from build123d import *

# Parameters (mm, degrees)
SKETCH_3_R                         = 2.75
EXTRUDE_1_DEPTH                    = 2
PATTERN_CIRCULAR_1_COUNT           = 4
SKETCH_7_R                         = 1.5
CUT_EXTRUDE_3_DEPTH                = 10
CUT_EXTRUDE_4_DEPTH                = 3
PATTERN_CIRCULAR_3_COUNT           = 3
PATTERN_CIRCULAR_3_ANGLE           = 60
PATTERN_CIRCULAR_4_COUNT           = 4
PATTERN_CIRCULAR_4_COPY_1_SKETCH_R = 1.5
PATTERN_CIRCULAR_4_COPY_1_DEPTH    = 10
PATTERN_CIRCULAR_4_COPY_2_SKETCH_R = 1.5
PATTERN_CIRCULAR_4_COPY_2_DEPTH    = 10
PATTERN_CIRCULAR_4_COPY_3_SKETCH_R = 1.5
PATTERN_CIRCULAR_4_COPY_3_DEPTH    = 10
PATTERN_CIRCULAR_4_COPY_4_SKETCH_R = 1.5
PATTERN_CIRCULAR_4_COPY_4_DEPTH    = 10
PATTERN_CIRCULAR_4_COPY_5_SKETCH_R = 1.5
PATTERN_CIRCULAR_4_COPY_5_DEPTH    = 10
PATTERN_CIRCULAR_4_COPY_6_SKETCH_R = 1.5
PATTERN_CIRCULAR_4_COPY_6_DEPTH    = 10
PATTERN_CIRCULAR_4_COPY_7_DEPTH    = 3
PATTERN_CIRCULAR_4_COPY_8_DEPTH    = 3
PATTERN_CIRCULAR_4_COPY_9_DEPTH    = 3
PATTERN_CIRCULAR_4_COPY_10_DEPTH   = 3
PATTERN_CIRCULAR_4_COPY_11_DEPTH   = 3
PATTERN_CIRCULAR_4_COPY_12_DEPTH   = 3
FILLET_1_R                         = 0.5


with BuildPart() as part:
    # 草图2 → 旋转1 (revolve)
    with BuildSketch(Plane(origin=(0, 0, 0), x_dir=(1, 0, 0), z_dir=(0, 1, 0)), mode=Mode.PRIVATE) as revolve_1_sk:
        Polygon((0, -2.5), (30, -2.5), (27.5, 0), (30, 2.5), (0, 2.5), align=None)
    revolve(revolve_1_sk.sketch.rotate(Axis((0, 0, -2.5), (0, 0, 1)), 180), axis=Axis((0, 0, -2.5), (0, 0, 1)))

    # 草图3 → 凸台-拉伸1 (add)
    with BuildSketch(Plane.XY.offset(2.5)):
        with Locations(Location((4.788152334, 17.869627786, 0), (0, 0, 180))):
            Circle(SKETCH_3_R)
    extrude_1 = extrude(amount=EXTRUDE_1_DEPTH)

    # 阵列(圆周)1: 凸台-拉伸1 ×4 about axis
    pattern_circular_1_axis = Axis((0, 0, 0), (0, 0, 1))
    for i in range(1, PATTERN_CIRCULAR_1_COUNT):
        add(extrude_1.rotate(pattern_circular_1_axis, i * 360 / PATTERN_CIRCULAR_1_COUNT))

    # 草图7 → 切除-拉伸3 (cut)
    with BuildSketch(Plane(origin=(0, 0, -2.5), x_dir=(-1, 0, 0), z_dir=(0, 0, -1))):
        with Locations((4.788152334, 17.869627786)):
            Circle(SKETCH_7_R)
    cut_extrude_3 = extrude(amount=-CUT_EXTRUDE_3_DEPTH, mode=Mode.SUBTRACT)

    # 草图8 → 切除-拉伸4 (cut)
    with BuildSketch(Plane(origin=(0, 0, -2.5), x_dir=(-1, 0, 0), z_dir=(0, 0, -1))):
        Polygon((3.966291485, 14.802401339), (7.033517932, 15.624262189), (7.855378781, 18.691488636), (5.610013184, 20.936854233), (2.542786737, 20.114993384), (1.720925887, 17.047766937), align=None)
    cut_extrude_4 = extrude(amount=-CUT_EXTRUDE_4_DEPTH, mode=Mode.SUBTRACT)

    # 阵列(圆周)3: 切除-拉伸3, 切除-拉伸4 ×3 about axis
    pattern_circular_3_axis = Axis((0, 0, 0), (0, 0, 1))
    add([cut_extrude_3.rotate(pattern_circular_3_axis, i * PATTERN_CIRCULAR_3_ANGLE / (PATTERN_CIRCULAR_3_COUNT - 1)) for i in range(1, PATTERN_CIRCULAR_3_COUNT)], mode=Mode.SUBTRACT)
    add([cut_extrude_4.rotate(pattern_circular_3_axis, i * PATTERN_CIRCULAR_3_ANGLE / (PATTERN_CIRCULAR_3_COUNT - 1)) for i in range(1, PATTERN_CIRCULAR_3_COUNT)], mode=Mode.SUBTRACT)

    # 阵列(圆周)4: 切除-拉伸3, 切除-拉伸4 ×4 about axis
    pattern_circular_4_axis = Axis((0, 0, 2.5), (0, 0, -1))
    add([cut_extrude_3.rotate(pattern_circular_4_axis, i * 360 / PATTERN_CIRCULAR_4_COUNT) for i in range(1, PATTERN_CIRCULAR_4_COUNT)], mode=Mode.SUBTRACT)
    add([cut_extrude_4.rotate(pattern_circular_4_axis, i * 360 / PATTERN_CIRCULAR_4_COUNT) for i in range(1, PATTERN_CIRCULAR_4_COUNT)], mode=Mode.SUBTRACT)

    # 阵列(圆周)4 copy 1 sketch → 阵列(圆周)4 copy 1 (cut)
    with BuildSketch(Plane(origin=(0, 0, -2.5), x_dir=(-0.5000000000000011, 0.866025403784438, 0), z_dir=(0, 0, -1))):
        with Locations((4.788152334, 17.869627786)):
            Circle(PATTERN_CIRCULAR_4_COPY_1_SKETCH_R)
    extrude(amount=-PATTERN_CIRCULAR_4_COPY_1_DEPTH, mode=Mode.SUBTRACT)

    # 阵列(圆周)4 copy 2 sketch → 阵列(圆周)4 copy 2 (cut)
    with BuildSketch(Plane(origin=(0, 0, -2.5), x_dir=(0.8660254037844379, 0.5000000000000012, 0), z_dir=(0, 0, -1))):
        with Locations((4.788152334, 17.869627786)):
            Circle(PATTERN_CIRCULAR_4_COPY_2_SKETCH_R)
    extrude(amount=-PATTERN_CIRCULAR_4_COPY_2_DEPTH, mode=Mode.SUBTRACT)

    # 阵列(圆周)4 copy 3 sketch → 阵列(圆周)4 copy 3 (cut)
    with BuildSketch(Plane(origin=(0, 0, -2.5), x_dir=(0.5000000000000012, -0.8660254037844379, 0), z_dir=(0, 0, -1))):
        with Locations((4.788152334, 17.869627786)):
            Circle(PATTERN_CIRCULAR_4_COPY_3_SKETCH_R)
    extrude(amount=-PATTERN_CIRCULAR_4_COPY_3_DEPTH, mode=Mode.SUBTRACT)

    # 阵列(圆周)4 copy 4 sketch → 阵列(圆周)4 copy 4 (cut)
    with BuildSketch(Plane(origin=(0, 0, -2.5), x_dir=(-0.8660254037844399, 0.4999999999999977, 0), z_dir=(0, 0, -1))):
        with Locations((4.788152334, 17.869627786)):
            Circle(PATTERN_CIRCULAR_4_COPY_4_SKETCH_R)
    extrude(amount=-PATTERN_CIRCULAR_4_COPY_4_DEPTH, mode=Mode.SUBTRACT)

    # 阵列(圆周)4 copy 5 sketch → 阵列(圆周)4 copy 5 (cut)
    with BuildSketch(Plane(origin=(0, 0, -2.5), x_dir=(0.49999999999999767, 0.86602540378444, 0), z_dir=(0, 0, -1))):
        with Locations((4.788152334, 17.869627786)):
            Circle(PATTERN_CIRCULAR_4_COPY_5_SKETCH_R)
    extrude(amount=-PATTERN_CIRCULAR_4_COPY_5_DEPTH, mode=Mode.SUBTRACT)

    # 阵列(圆周)4 copy 6 sketch → 阵列(圆周)4 copy 6 (cut)
    with BuildSketch(Plane(origin=(0, 0, -2.5), x_dir=(0.86602540378444, -0.4999999999999976, 0), z_dir=(0, 0, -1))):
        with Locations((4.788152334, 17.869627786)):
            Circle(PATTERN_CIRCULAR_4_COPY_6_SKETCH_R)
    extrude(amount=-PATTERN_CIRCULAR_4_COPY_6_DEPTH, mode=Mode.SUBTRACT)

    # 阵列(圆周)4 copy 7 sketch → 阵列(圆周)4 copy 7 (cut)
    with BuildSketch(Plane(origin=(0, 0, -2.5), x_dir=(-0.5000000000000011, 0.866025403784438, 0), z_dir=(0, 0, -1))):
        Polygon((3.966291485, 14.802401339), (7.033517932, 15.624262189), (7.855378781, 18.691488636), (5.610013184, 20.936854233), (2.542786737, 20.114993384), (1.720925887, 17.047766937), align=None)
    extrude(amount=-PATTERN_CIRCULAR_4_COPY_7_DEPTH, mode=Mode.SUBTRACT)

    # 阵列(圆周)4 copy 8 sketch → 阵列(圆周)4 copy 8 (cut)
    with BuildSketch(Plane(origin=(0, 0, -2.5), x_dir=(0.8660254037844379, 0.5000000000000012, 0), z_dir=(0, 0, -1))):
        Polygon((3.966291485, 14.802401339), (7.033517932, 15.624262189), (7.855378781, 18.691488636), (5.610013184, 20.936854233), (2.542786737, 20.114993384), (1.720925887, 17.047766937), align=None)
    extrude(amount=-PATTERN_CIRCULAR_4_COPY_8_DEPTH, mode=Mode.SUBTRACT)

    # 阵列(圆周)4 copy 9 sketch → 阵列(圆周)4 copy 9 (cut)
    with BuildSketch(Plane(origin=(0, 0, -2.5), x_dir=(0.5000000000000012, -0.8660254037844379, 0), z_dir=(0, 0, -1))):
        Polygon((3.966291485, 14.802401339), (7.033517932, 15.624262189), (7.855378781, 18.691488636), (5.610013184, 20.936854233), (2.542786737, 20.114993384), (1.720925887, 17.047766937), align=None)
    extrude(amount=-PATTERN_CIRCULAR_4_COPY_9_DEPTH, mode=Mode.SUBTRACT)

    # 阵列(圆周)4 copy 10 sketch → 阵列(圆周)4 copy 10 (cut)
    with BuildSketch(Plane(origin=(0, 0, -2.5), x_dir=(-0.8660254037844399, 0.4999999999999977, 0), z_dir=(0, 0, -1))):
        Polygon((3.966291485, 14.802401339), (7.033517932, 15.624262189), (7.855378781, 18.691488636), (5.610013184, 20.936854233), (2.542786737, 20.114993384), (1.720925887, 17.047766937), align=None)
    extrude(amount=-PATTERN_CIRCULAR_4_COPY_10_DEPTH, mode=Mode.SUBTRACT)

    # 阵列(圆周)4 copy 11 sketch → 阵列(圆周)4 copy 11 (cut)
    with BuildSketch(Plane(origin=(0, 0, -2.5), x_dir=(0.49999999999999767, 0.86602540378444, 0), z_dir=(0, 0, -1))):
        Polygon((3.966291485, 14.802401339), (7.033517932, 15.624262189), (7.855378781, 18.691488636), (5.610013184, 20.936854233), (2.542786737, 20.114993384), (1.720925887, 17.047766937), align=None)
    extrude(amount=-PATTERN_CIRCULAR_4_COPY_11_DEPTH, mode=Mode.SUBTRACT)

    # 阵列(圆周)4 copy 12 sketch → 阵列(圆周)4 copy 12 (cut)
    with BuildSketch(Plane(origin=(0, 0, -2.5), x_dir=(0.86602540378444, -0.4999999999999976, 0), z_dir=(0, 0, -1))):
        Polygon((3.966291485, 14.802401339), (7.033517932, 15.624262189), (7.855378781, 18.691488636), (5.610013184, 20.936854233), (2.542786737, 20.114993384), (1.720925887, 17.047766937), align=None)
    extrude(amount=-PATTERN_CIRCULAR_4_COPY_12_DEPTH, mode=Mode.SUBTRACT)

    # 圆角1
    fillet_1_edges = [part.edges().sort_by_distance(p)[0] for p in [
        (30, 0, -2.5),
        (30, 0, 2.5),
    ]]
    fillet(fillet_1_edges, radius=FILLET_1_R)


solid = part.part
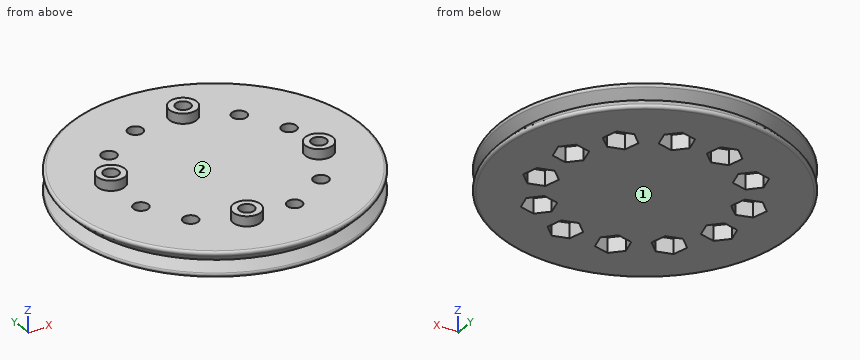
Geometry: final body of the model. Coordinates: model frame, mm. Face numbers are marked on the shaded views. A direction names the side the tool comes from. Coordinates: 2 decimals unless noted, no trailing zeros. Order: outer loops, then holes, each group sorted by start corner. A loop starts at its lowest first (then second) coordinate and runs counter-clockwise, first axis right, second up. Notation, with made-up numbers: (50, 10) - (88, 10) arc R27 ccw to (88, 31) - close; hole circle Ø5 at (82, 64.25). An arc over 180 degrees is marked (long way). Use one line per item in the form item = value.
1) Section A-A (x = 0). Return loops of the section in (y, z), then the cut area to 3 significant figures.
Solutions:
outline = (-29.15, -1.65) arc R0.5 ccw to (-28.79, -2.5) - (28.79, -2.5) arc R0.5 ccw to (29.15, -1.65) - (27.5, 0) - (29.15, 1.65) arc R0.5 ccw to (28.79, 2.5) - (-28.79, 2.5) arc R0.5 ccw to (-29.15, 1.65) - (-27.5, 0) - close
area = 286 mm^2
2) Pin query (flat end, axial travel): pin 1 (5 mm diameter, centred on x = -17.87, y = -4.79, fed in from -Z); pin 2 (3 mm diameter, centred on x = 13.5, z = 3.5, fed in from -Y); pin 3 (3.5 mm diameter, centred on x = 4.79, y = -17.87, fed in from +Z). Return the tip coordinate at first contact, or that it passes through.
Solutions:
pin_1 = 0.5
pin_2 = -26.34
pin_3 = 2.5
3) Ray query, L1, parallel to X at y = -17.5, z = 1; L2, parallel to X at y = 6.5, z = -1.5; L3, parallel to Y at x = -3, z = -0.5. Return the intervals inside material, ascending.
Solutions:
L1 = -22.49 to -6.24, -3.33 to 3.33, 6.24 to 22.49
L2 = -28.26 to -20.05, -15.48 to 15.48, 20.05 to 28.26
L3 = -27.84 to -20.24, -15.77 to 15.77, 20.24 to 27.84
4) Set-up query: the marked faces 1 and 2. Return all of +Z, -Z, +X, -X, +Y, -Y with unobstructed straight access to the full face (end or side cutting, diameter ignored); none if empty.
Solutions:
face_1 = -Z, +X, -X, +Y, -Y
face_2 = +Z
